Could you check a few things on this model? Use its own coordinates, in mm. A direction names the side the tool comes from. Coordinates: 2 decimals unless noted, no trailing zeros. Order: outer loops, then holes, each group sorted by start corner. A loop starts at its lowest first (then second) coordinate and runs counter-clockwise, first axis right, second up. Notation, with made-up numbers: (-30.5, -33) - (-18.5, -33) arc R20 ccw to (-18.5, 3) - close; hole circle Ø7 at (-18, -32). An arc over 180 degrees is marked (long way). One line per item, written item: value.
from build123d import *

# Parameters (mm, degrees)
SKETCH1_R           = 7.5
BOSS_EXTRUDE1_DEPTH = 5
BOSS_EXTRUDE2_DEPTH = 5
BOSS_EXTRUDE2_TAPER = 3
SKETCH3_R           = 4
BOSS_EXTRUDE3_DEPTH = 10


with BuildPart() as part:
    # Sketch1 → Boss-Extrude1 (new body)
    with BuildSketch(Plane(origin=(0, 0, 0), x_dir=(1, 0, 0), z_dir=(0, 1, 0))):
        with Locations(Location((0, 0, 0), (0, 0, 270))):
            Circle(SKETCH1_R)
    extrude(amount=BOSS_EXTRUDE1_DEPTH)

    # Sketch2 → Boss-Extrude2 (add)
    with BuildSketch(Plane(origin=(0, 5, 0), x_dir=(1, 0, 0), z_dir=(0, 1, 0))):
        Polygon((0, 5.773502692), (-5, -2.886751346), (5, -2.886751346), align=None)
    extrude(amount=BOSS_EXTRUDE2_DEPTH, taper=BOSS_EXTRUDE2_TAPER)

    # Sketch3 → Boss-Extrude3 (add)
    with BuildSketch(Plane.XZ):
        with Locations(Location((0, 0, 0), (0, 0, 270))):
            Circle(SKETCH3_R)
    extrude(amount=BOSS_EXTRUDE3_DEPTH)


solid = part.part
Item 1: I want a section at D-D on z = 5.5. Please give me the cut outline in (x, y).
Conclusion:
outline: (-5.1, 0) - (5.1, 0) - (5.1, 5) - (-5.1, 5) - close
Item 2: If I drill on probe 1 along Y at (x, z) = (3.25, -6); probe 2 along Y at (x, z) = (0.25, 3.25); probe 3 along X at (y, z) = (4.5, -4.5), over which ranges is the centre line in solid material (lowest first)?
Conclusion:
probe 1: 0 to 5
probe 2: -10 to 5
probe 3: -6 to 6
Item 3: I'm going to push flat-ended pins straight in: pin 1 Ø6 at (x, y) = (2, -6) entering from +Z; pin 2 Ø1.5 at (y, z) = (5.5, 3.5) entering from +X; pin 3 Ø2 at (x, z) = (5, 2.5) entering from +Y; pin 4 Ø2 at (y, z) = (-2, 4) entering from +X. Where does each tip first touch, or does it pass through?
Conclusion:
pin 1: z = 4
pin 2: x = 6.9
pin 3: y = 10
pin 4: x = 2.65
Item 4: I want a section at A-A on y = 1.75. Please give me the cut outline in (x, z), then the cut area to 3 significant figures.
Conclusion:
outline: circle Ø15 at (0, 0)
area: 177 mm²
Item 5: I want a section at C-C on y = -1.25. Please give me the cut outline in (x, z), then the cut area to 3 significant figures.
Conclusion:
outline: circle Ø8 at (0, 0)
area: 50.3 mm²
Item 6: I want a section at B-B on x = -5.5. Please give me the cut outline in (y, z).
Conclusion:
outline: (0, -5.1) - (5, -5.1) - (5, 5.1) - (0, 5.1) - close
Item 7: For faces 1 (the face through (0.33, 2.465, -7.493)), 2 (the face through (-3.905, -4.93, 0.867)), 3 (the face through (0.1, 5, 3.2)), which set-ups out of +Z, -Z, +X, -X, +Y, -Y let a thin tool reach every point of the face, with its end or its side?
Conclusion:
face 1: +Y, -Y
face 2: -Y
face 3: +Y
